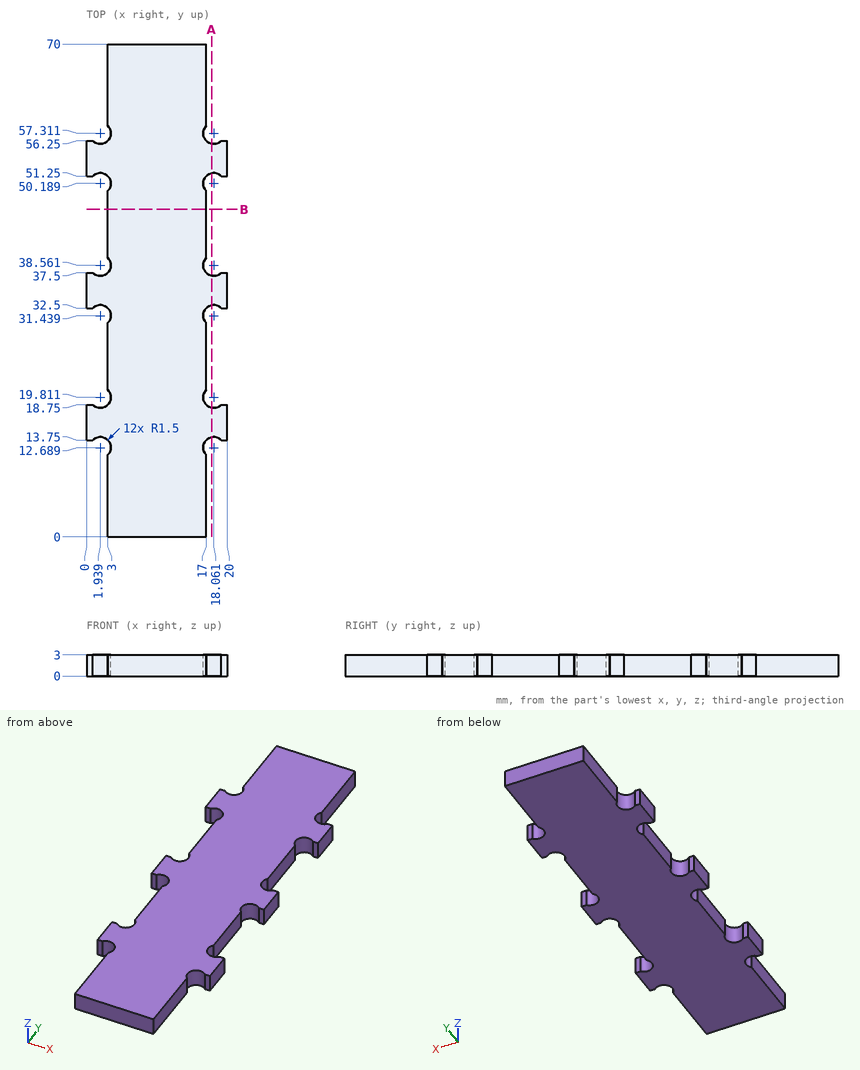
Print and shaded views of the part. All mm, measured from the part's lowest x, y and z. Give positions to 0.01 mm unless a question says otherwise; leave off trailing zeros. Loops run counter-clockwise (first coordinate to the right, second up) from the corner with the lowest first, then second, coordinate; pieces in that order, holes last. Notation, with made-up numbers: (74.5, 73) -> (114.5, 73) arc R15 ccw to (114.5, 88) -> close; hole circle Ø8 at (29.25, 5). An arc over 180 degrees is marked (long way). Use a Markdown table: item, result.
1. Wall check: L1, parallel to Y at x = 18.5, z = 2.55; L2, parallel to Y at x = 17.25, z = 0.55; L3, parallel to X at y = 61.5, z = 2. Give the ranges that are in metal, low to high. Write a range as [from, to].
Check result:
| item | result |
|---|---|
| L1 | y = [14.12, 18.38], [32.87, 37.13], [51.62, 55.88] |
| L2 | y = [13.95, 18.55], [32.7, 37.3], [51.45, 56.05] |
| L3 | x = [3, 17] |
2. Flat gauge pins, fed straight in: pin 1 (1 mm diameter, centred on x = 19.5, z = 2, fed in from -Y); pin 2 (1 mm diameter, centred on y = 22, z = 1, fed in from +X); pin 3 (1.5 mm diameter, centred on y = 7, z = 1.5, fed in from -X). Where does each tip first touch, or does it go through?
Check result:
| item | result |
|---|---|
| pin 1 | stops at y = 13.75 |
| pin 2 | stops at x = 17 |
| pin 3 | stops at x = 3 |
3. Slice it at B-B (y = 46.5). List the corners of the cut face in (x, z).
Check result:
| item | result |
|---|---|
| outline | (3, 0) -> (17, 0) -> (17, 3) -> (3, 3) -> close |
4. Slice it at A-A (x = 17.75). List the corners of the cut face in (y, z).
Check result:
| item | result |
|---|---|
| outline | (14.16, 0) -> (18.34, 0) -> (18.34, 3) -> (14.16, 3) -> close; (32.91, 0) -> (37.09, 0) -> (37.09, 3) -> (32.91, 3) -> close; (51.66, 0) -> (55.84, 0) -> (55.84, 3) -> (51.66, 3) -> close |
